The drawing under review shows one solid part. Ordinate dimensions are in mm from its lowest x, y, z. A direction names the side the tool comes from. Round coordinates to 2 decimals unless told otherwise and drop trailing zeros. Order: outer loops, then holes, each group sorted by start corner. A loop starts at its lowest first (then second) coordinate and runs counter-clockwise, first axis right, second up.
1) Mouldability with a two-part tool opening along Z and no side actions: class the marked faces 4, 5 and 6 as pulls with the +Z half, pulls with the -Z half, needs draft (parallel to the pull), parting line crosses it, or undercut.
2) Machinability: for the marked faces 1, 2 and 3, which of the approach directions +Z, -Z, +X, -X, +Y, -Y give a long, thin tool a straight path to every point of the face, cutting with its end or side? Answer none if there is none.
3) Clearance check with flat-ended pins moving along their axes: P1, Ø6, axis at x = 16.5, z = 28, coming from the -Y side; P2, Ø11, axis at y = 42, z = 7.5, coming from the +X side. State where each tip first meets the part, or that it passes through.
4) To check wall thickness, follow L1, parallel to X at y = 34.5, z = 37; L2, parallel to Z at x = 25, y = 19 (3 decimals); L3, parallel to Z at x = 61.5, y = 42. State the ranges of each line that lie inside material, in increasing order.
5) Consider section A-A (z = 9). Give the boundary of the cut face in (x, y), then the cut area to 3 significant figures.
6) Consider section B-B (x = 46.5). Give the boundary of the cut face in (y, z).
7) Consider section C-C (y = 40.5). Give the boundary of the cut face in (x, z), then the cut area to 3 significant figures.
8) Consider section D-D (z = 37). Give the boundary of the cut face in (x, y).
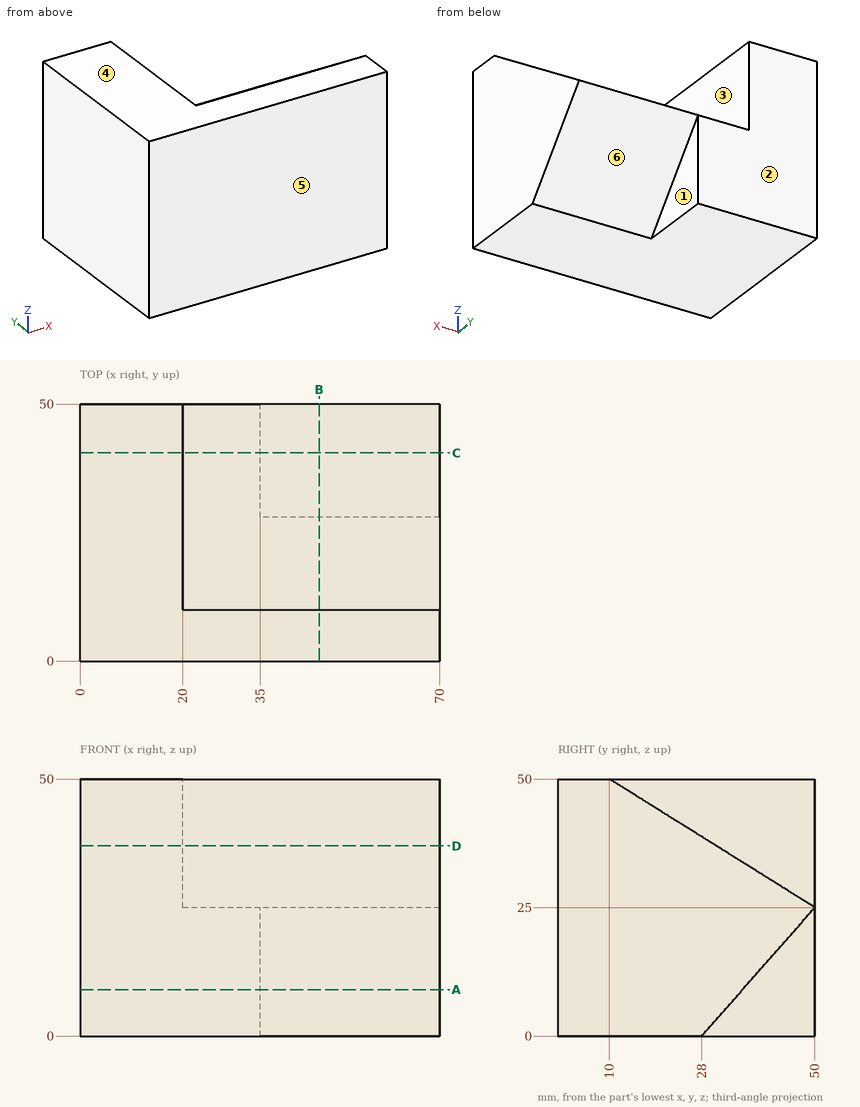
Answer below:
1. face 4: pulls with the +Z half
1. face 5: needs draft
1. face 6: pulls with the -Z half
2. face 1: -Z, +X, +Y
2. face 2: +Z, -Z, +X, -X, +Y
2. face 3: +Z, +X, +Y
3. P1: stops at y = 0
3. P2: stops at x = 35
4. L1: x = 0 to 20
4. L2: z = 0 to 44.375
4. L3: z = 15.91 to 30
5. outline: (0, 0) - (70, 0) - (70, 35.92) - (35, 35.92) - (35, 50) - (0, 50) - close
5. area: 3,010 mm2
6. outline: (0, 0) - (28, 0) - (50, 25) - (10, 50) - (0, 50) - close
7. outline: (0, 0) - (35, 0) - (35, 14.2) - (70, 14.2) - (70, 30.94) - (20, 30.94) - (20, 50) - (0, 50) - close
7. area: 2,050 mm2
8. outline: (0, 0) - (70, 0) - (70, 30.8) - (20, 30.8) - (20, 50) - (0, 50) - close
